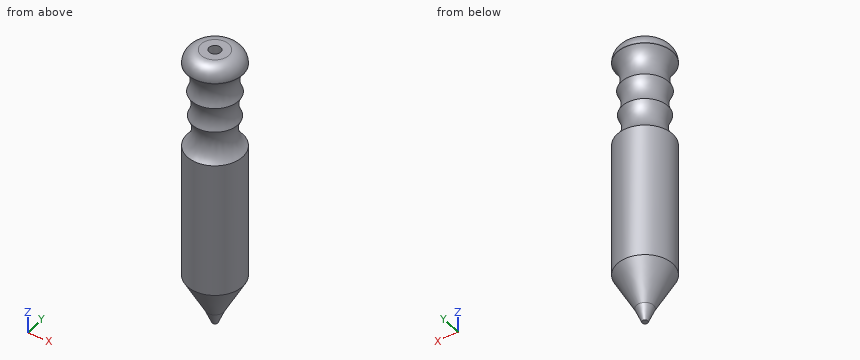
from build123d import *

# Parameters (mm, degrees)
F2_R = 5


with BuildPart() as f1:
    # F0 (on Front) → F1 (revolve)
    with BuildSketch(Plane.XZ):
        with BuildLine():
            Line((-3.074385, 5), (-1, 0))
            Line((-1, 0), (0, 0))
            Line((0, 0), (0, 17.69474))
            Line((0, 17.69474), (-2.1, 17.69474))
            Line((-2.1, 17.69474), (-2.1, 102.69474))
            Line((-2.1, 102.69474), (-10, 102.69474))
            Line((-10, 102.69474), (-10, 97.513927))
            ThreePointArc((-10, 97.513927), (-7.529704, 92.507199), (-8.497441, 87.00873))
            ThreePointArc((-8.497441, 87.00873), (-7.145288, 82.498591), (-8.262521, 77.924594))
            ThreePointArc((-8.262521, 77.924594), (-7.078613, 71.935289), (-10, 66.574422))
            Line((-10, 66.574422), (-10, 17.69474))
            Line((-10, 17.69474), (-3.074385, 5))
        make_face()
    revolve(axis=Axis((0, 0, 8.84737), (0, 0, -1)))

    # F2
    f2_edges = [f1.edges().sort_by_distance(p)[0] for p in [
        (10, 0, 102.69474),
    ]]
    fillet(f2_edges, radius=F2_R)


solid = f1.part
The listing builds one solid part. Answer for the finished solid, in the listing's coordinates (mm). Coordinates: 2 decimals unless noted, no trailing zeros. Loops run counter-clockwise (first coordinate to the right, second up) from the corner with the lowest first, then second, coordinate; pieces in that order, holes last. Notation, with made-up numbers: M 6.5,44.25 L 20.5,44.25 A5 ccw 20.5,50.25 Z; hole C 61,8.5 d4. An arc over 180 degrees is marked long. Answer in a Markdown table with one row per item.
1) Given pin 1 (8 mm diameter, centred on x = -7, z = 86, fed in from -Y); pin 2 (6 mm diameter, centred on x = 2, z = 18, fed in from -Y); pin 3 (6 mm diameter, centred on y = -6, z = 81.5, fed in from -X); pin 4 (1 mm diameter, centred on x = -6, z = 87, fed in from -Y), each flat-ended and moving along its own axis, determine where each tip first touches the part or whether it passes through.
Answers below:
| item | result |
|---|---|
| pin 1 | y = -7.9 |
| pin 2 | y = -10 |
| pin 3 | x = -6.61 |
| pin 4 | y = -6.48 |
2) Find the intervals of material crossed by probe 1 along Y at (x, z) = (0, 60); probe 2 along Z at (x, y) = (-5.25, 6.5); probe 3 along X at (y, z) = (-1, 43.5), in increasing order.
Answers below:
| item | result |
|---|---|
| probe 1 | -10 to -2.1, 2.1 to 10 |
| probe 2 | 14.68 to 68.51, 86.77 to 87.29, 95.19 to 101.4 |
| probe 3 | -9.95 to -1.85, 1.85 to 9.95 |
3) Find section A-A (z = 36). Determine the outline of the cut face in (x, y), then the cut area to 3 significant figures.
Answers below:
| item | result |
|---|---|
| outline | C 0,0 d20; hole C 0,0 d4.2 |
| area | 300 mm^2 |
